Check sheet for the drawn part. Datum: minimum x, y, z corner. Units: mm. A direction names the side the tool comes from. Round coordinates to 2 decimals unless told otherwise and drop trailing zeros. Loops run counter-clockwise (first coordinate to the right, second up) from the corner with the lowest first, then second, coordinate; pieces in that order, holes last.
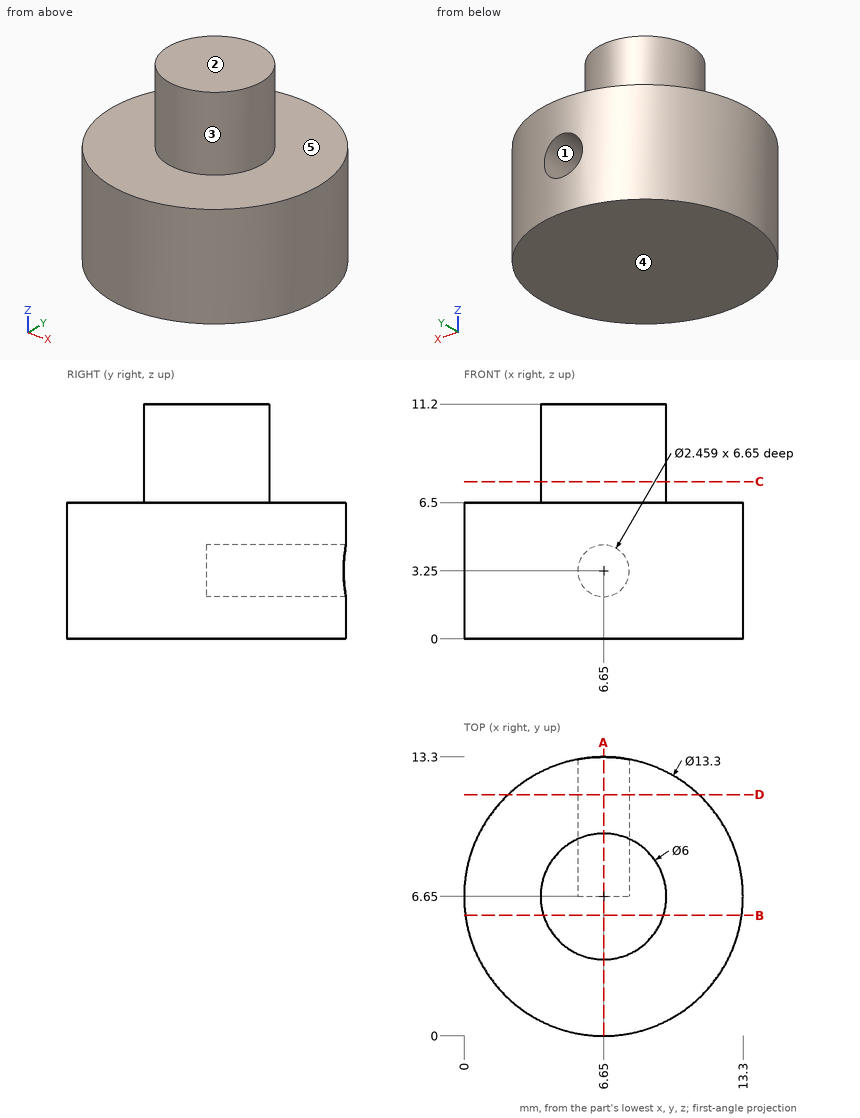
1) Access from +Z, -Z, +X, -X, +Y, -Y to the whole of each face (thin tool, end or side, straight path). Record for the marked faces 4 and 5.
Report:
face 4: -Z, +X, -X, +Y, -Y
face 5: +Z
2) Sectioned sample at C-C, the plane z = 7.5. Record the cut outline in (x, y).
Report:
outline: circle Ø6 at (6.65, 6.65)
3) Sectioned sample at A-A, the plane x = 6.65. Record the cut outline in (y, z), then the cut area to 3 significant figures.
Report:
outline: (0, 0) - (13.3, 0) - (13.3, 2.02) - (6.65, 2.02) - (6.65, 4.48) - (13.3, 4.48) - (13.3, 6.5) - (9.65, 6.5) - (9.65, 11.2) - (3.65, 11.2) - (3.65, 6.5) - (0, 6.5) - close
area: 98.3 mm2
4) Gauge pin test, flat ends, axial feed: pin 1 (3 mm diameter, centred on x = 8, z = 2.5, fed in from +Y); pin 2 (4 mm diameter, centred on x = 11, z = 2, fed in from +Y); pin 3 (0.7 mm diameter, centred on x = 6.5, z = 3, fed in from +Y); pin 4 (1.5 mm diameter, centred on y = 8, z = 8.5, fed in from -X). Record the tip position at first contact, or that the pin passes through.
Report:
pin 1: stops at y = 13.3
pin 2: stops at y = 12.87
pin 3: stops at y = 6.65
pin 4: stops at x = 3.71
5) Sectioned sample at D-D, the plane y = 11.5. Record the cut outline in (x, z), then the cut area to 3 significant figures.
Report:
outline: (2.1, 0) - (11.2, 0) - (11.2, 6.5) - (2.1, 6.5) - close; hole circle Ø2.46 at (6.65, 3.25)
area: 54.4 mm2
6) Sectioned sample at B-B, the plane y = 5.75. Record the cut outline in (x, z).
Report:
outline: (0.06, 0) - (13.24, 0) - (13.24, 6.5) - (9.51, 6.5) - (9.51, 11.2) - (3.79, 11.2) - (3.79, 6.5) - (0.06, 6.5) - close
7) Scan lines: line 1 along Z through (x, y) = (11, 9); line 2 along X through (y, z) = (5, 7.25); line 3 along Y through (x, z) = (11, 1). Record each from-to range of solid material in increasing order.
Report:
line 1: z = 0 to 6.5
line 2: x = 4.14 to 9.16
line 3: y = 1.62 to 11.68
8) Mould release check, pull along Z, two halves, no side actions. Record for the marked faces 1, 2 and 3: +Z half, -Z half, draft (parallel to the pull), parting line (faces both ways), or undercut.
Report:
face 1: undercut
face 2: +Z half
face 3: draft
